The model under review builds one solid part; all positions refer to its coordinate system, in mm. A direction names the side the tool comes from. Coordinates: 2 decimals unless noted, no trailing zeros. Order: outer loops, then holes, each group sorted by start corner. A loop starts at its lowest first (then second) coordinate and runs counter-clockwise, first axis right, second up. Notation, with made-up numbers: M 44.5,0 L 83.5,0 A19 ccw 83.5,13 Z; hole C 54,70.25 d4. An arc over 180 degrees is marked long. Answer as CSV lines item,"result". Start each with the question number.
Q1. The part is to be moulded in two halves that separate along Z. For faces 3 (the face through (-19, 36, 3)), 4 (the face through (0, 34, 2.2)), 5 (the face through (0, 35, 0)), say which applies: +Z half, -Z half, draft (parallel to the pull), parting line (faces both ways), or undercut.
Q2. Consider section C-C on y = 35. Write out the cut boundary in (x, z).
Q3. Consider section B-B on x = -15. Write out the cut boundary in (y, z), and give its area (3 significant figures).
Q4. Consider section A-A on z = 5.55. Write out the cut boundary in (x, y), and give its area (3 significant figures).
Q5. Machinability: for faces 1 (the face through (0, 39, 3)), 2 (the face through (17.661, 33.646, 3.186)), which of the approach directions +Z, -Z, +X, -X, +Y, -Y give a long, thin tool a straight path to every point of the face, cutting with its end or side? Answer none if there is none.
Q6. Wall thickness on L1, parallel to Z at x = -7, y = 34; L2, parallel to X at y = 35.5, z = 1.8; L3, parallel to Y at x = 15, z = 1.6: over which ranges is each line inside the solid? List them lowest first. Write a range as [from, to].
Q7. Consider section D-D on z = 2.6. Write out the cut boundary in (x, y).
from build123d import *

# Parameters (mm, degrees)
CYLINDER028_R     = 38
CYLINDER028_DEPTH = 2
CYLINDER031_R     = 1.5
CYLINDER031_DEPTH = 10
CYLINDER032_R     = 1.5
CYLINDER032_DEPTH = 10
BOX033_W          = 38
BOX033_H          = 8
BOX033_DEPTH      = 6
FILLET006_R       = 1.6


with BuildPart() as cylinder007:
    # Cylinder028 → Cylinder028 (new body)
    with BuildSketch(Plane.XY.offset(2.2)):
        Circle(CYLINDER028_R)
    extrude(amount=CYLINDER028_DEPTH)


with BuildPart() as cylinder010:
    # Cylinder031 → Cylinder031 (new body)
    with BuildSketch(Plane(origin=(-15, -35, 0), x_dir=(1, 0, 0), z_dir=(0, 0, 1))):
        Circle(CYLINDER031_R)
    extrude(amount=CYLINDER031_DEPTH)


with BuildPart() as fusion017:
    # Cylinder032 → Cylinder032 (new body)
    with BuildSketch(Plane(origin=(15, -35, 0), x_dir=(1, 0, 0), z_dir=(0, 0, 1))):
        Circle(CYLINDER032_R)
    extrude(amount=CYLINDER032_DEPTH)

    # Fusion017: union Cylinder010
    add(cylinder010.part)


with BuildPart() as cut031:
    # Box033 → Box033 (new body)
    with BuildSketch(Plane(origin=(-19, -39, 0), x_dir=(1, 0, 0), z_dir=(0, 0, 1))):
        with Locations((19, 4)):
            Rectangle(BOX033_W, BOX033_H)
    extrude(amount=BOX033_DEPTH)

    # Fillet006
    fillet006_edges = [cut031.edges().sort_by_distance(p)[0] for p in [
        (-19, -31, 3),
        (19, -31, 3),
    ]]
    fillet(fillet006_edges, radius=FILLET006_R)

    # Cut030: cut Fusion017
    add(fusion017.part, mode=Mode.SUBTRACT)

    # Cut031: cut Cylinder007
    add(cylinder007.part, mode=Mode.SUBTRACT)


with BuildPart() as part_mirroring003:
    # Part__Mirroring003: instance of Cut031
    add(cut031.part.mirror(Plane(origin=(0, 0, 0), x_dir=(1, 0, 0), z_dir=(0, 1, 0))))


solid = part_mirroring003.part
Evaluation:
1,face 3,"draft"
1,face 4,"undercut"
1,face 5,"-Z half"
2,outline,"M -19,0 L -16.5,0 L -16.5,6 L -19,6 Z; M -13.5,0 L 13.5,0 L 13.5,2.2 L -13.5,2.2 Z; M -13.5,4.2 L 13.5,4.2 L 13.5,6 L -13.5,6 Z; M 16.5,0 L 19,0 L 19,6 L 16.5,6 Z"
3,outline,"M 31,0 L 33.5,0 L 33.5,2.2 L 31,2.2 Z; M 31,4.2 L 33.5,4.2 L 33.5,6 L 31,6 Z; M 36.5,0 L 39,0 L 39,6 L 36.5,6 Z"
3,area,"25.0 mm²"
4,outline,"M -19,32.6 A1.6 ccw -17.4,31 L 17.4,31 A1.6 ccw 19,32.6 L 19,39 L -19,39 Z; hole C -15,35 d3; hole C 15,35 d3"
4,area,"289 mm²"
5,face 1,"+Z, -Z, +X, -X, +Y"
5,face 2,"-Y"
6,L1,"z = [0, 2.2], [4.2, 6]"
6,L2,"x = [-19, -16.41], [-13.59, 13.59], [16.41, 19]"
6,L3,"y = [31, 33.5], [36.5, 39]"
7,outline,"M -19,32.91 A38 cw -16.33,34.31 A1.5 cw long -13.58,35.49 A38 cw 13.58,35.49 A1.5 cw long 16.33,34.31 A38 cw 19,32.91 L 19,39 L -19,39 Z"
